Could you check a few things on this model? Use its own coordinates, in mm. Face numbers are marked on the shaded views. Coordinates: 2 decimals unless noted, no trailing zeros. Loops run counter-clockwise (first coordinate to the right, second up) from the corner with the lowest first, then second, coordinate; pieces in that order, holes last. Notation, with made-up numbers: (49.5, -33.75) -> (59.5, -33.75) arc R3 cw to (59.5, -28.75) -> close; hole circle Ø6 at (70, 33). An arc over 180 degrees is marked (long way). One line per question, with ' | ' between items.
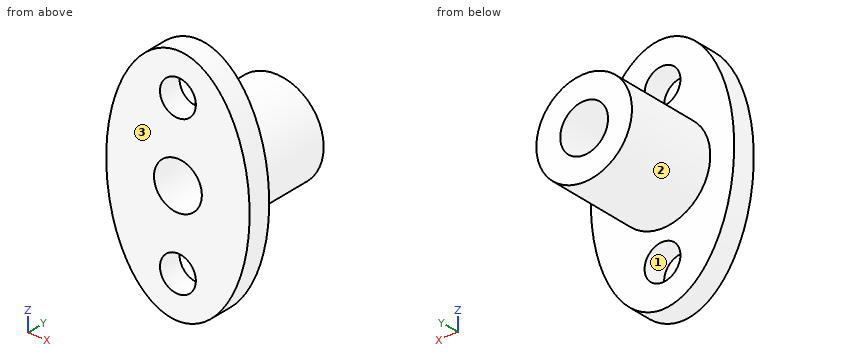
Autodesk Inventor part; units mm, degrees
ref_plane "YZ Plane" through (0, 0, 0) normal (1, 0, 0) x (0, 1, 0)
ref_plane "XZ Plane" through (0, 0, 0) normal (0, 1, 0) x (-1, 0, 0)
ref_plane "XY Plane" through (0, 0, 0) normal (0, 0, 1) x (1, 0, 0)
sketch "Sketch3" plane through (0, 0, 0) normal (0, 1, 0) x (-1, 0, 0)
  ellipse E0 centre (0, 0) end of major axis (0, -10) minor radius 6
  circle A0 centre (0, 0) radius 2
  circle A1 centre (0, 6.5026) radius 1.5
  circle A2 centre (0, -6.5) radius 1.5
  dimension "d0" = 6
  dimension "d3" = 10
  dimension "d2" = 4
  dimension "d5" = 3
  dimension "d9" = 6.5026
  dimension "d11" = 3
  dimension "d12" = 6.5
extrude "Extrusion1" add sketch "Sketch3" along normal blind 2
sketch "Sketch4" plane through (0, 2, 0) normal (0, 1, 0) x (1, 0, 0)
  circle A0 centre (0, 0) radius 4
  circle A1 centre (0, 0) radius 2
  dimension "d15" = 8
  dimension "d16" = 4
extrude "Extrusion2" add sketch "Sketch4" along normal blind 8
properties part number "reverse gear blands"
Q1. Imagine slicing it at B-B on y = 4.75. Write out the boundary of the cut face in (x, z), plus the area to 3 significant figures.
Values follow:
outline: circle Ø8 at (0, 0); hole circle Ø4 at (0, 0) | area: 37.7 mm2
Q2. Please list where these lines run through material, in increasing order: L1, parallel to Z at x = 0, y = 1.6; L2, parallel to Z at x = 0, y = 4.25. Write a range as [from, to].
Values follow:
L1: z = [-10, -8], [-5, -2], [2, 5], [8, 10] | L2: z = [-4, -2], [2, 4]
Q3. For pin 1 (1 mm diameter, centred on x = -3.5, z = -5.5, fed in from -Y); pin 2 (6 mm diameter, centred on y = 8.5, z = -5, fed in from +X); pin 3 (6 mm diameter, centred on x = -4.5, y = 2.5, fed in from -Z); pin 4 (4 mm diameter, centred on x = 0, z = -6.5, fed in from +Y), each with a flat end and sliding along its axis, tell me the tip position at first contact or that it passes through.
Values follow:
pin 1: stops at y = 0 | pin 2: stops at x = 3.46 | pin 3: stops at z = -9.66 | pin 4: stops at y = 2
Q4. We'd pull the mould along Z, two halves only. Please class the marked faces 1, 2 and 3: released by +Z, released by -Z, zero draft, split by the parting line, or undercut.
Values follow:
face 1: undercut | face 2: split by the parting line | face 3: zero draft
